Can you work these out from the model? Positions are in its coordinate system, mm. A direction names the side the tool comes from. Give positions to 0.01 mm unless a question says otherwise; leave off trailing zeros. Order: outer loops, then holes, each group sorted by start corner. A loop starts at its lowest first (then second) coordinate and runs counter-clockwise, first axis right, second up.
Item 1: If we mould it in two halves opening along Y, with no side actions, what happens to faces 1 (the flat face through (-47.1, 62, 1)), 2 (the flat face through (39.8, 61.57, 1.48)), 3 (the flat face through (-42, 66.1, 1)), 4 (the flat face through (-71, 3, 1))? For each: +Y half, -Y half, draft (parallel to the pull), parting line (faces both ways), or undercut.
Item 2: I want a section at A-A, the plane x = -69.5. Write out the boundary of the cut face in (y, z), then the cut area to 3 significant figures.
Item 3: Which directions (+Z, -Z, +X, -X, +Y, -Y) give clear straight access to the entire face, cutting with the end or side of a thin tool? Please do faces 5 (the flat face through (-50.2, 61.57, 1.48)), 6 (the flat face through (-56.056, -2.735, 1.479)), 7 (the flat face through (-52.1, 59, 1)).
Item 4: If I drill on line 1 along X through (y, z) = (63, 2.45); line 2 along X through (y, z) = (57.5, 2.75); line 3 along Y through (x, z) = (32, 1), over which ranges is the centre line in solid material (lowest first)?
Item 5: I'm going to push flat-ended pins straight in: pin 1 Ø1.5 at (x, z) = (60, 1) entering from -Y; pin 2 Ø8 at (x, y) = (-14, 10.5) entering from -Z; pin 3 Ø1.5 at (y, z) = (2, 1.5) entering from -X; pin 4 Ø0.9 at (y, z) = (2, 1.5) entering from +X. Where does each tip first touch, or does it pass through?
```python
from build123d import *

# Parameters (mm, degrees)
SKETCH1_W            = 162.421633227
SKETCH1_H            = 57
BOSS_EXTRUDE1_DEPTH  = 3
BOTTOM_HOOKS_DEPTH   = 3
TOP_TABS_DEPTH       = 3
TOP_TAB_RELIEF_REACH = 107.556


with BuildPart() as part:
    # Sketch1 → Boss-Extrude1 (new body)
    with BuildSketch(Plane.XY):
        with Locations((-1.032340883, 31.5)):
            Rectangle(SKETCH1_W, SKETCH1_H)
    extrude(amount=BOSS_EXTRUDE1_DEPTH)

    # Sketch2 → bottom hooks (add)
    with BuildSketch(Plane(origin=(0, 0, 0), x_dir=(-1, 0, 0), z_dir=(0, 0, -1))):
        Polygon((52, 3), (60, 3), (60, -0.2), (63, -0.2), (63, -2.2), (65, -2.2), (65, -5.2), (60, -5.2), (52, -0.2), align=None)
        Polygon((-53, -2.2), (-55, -2.2), (-55, -5.2), (-45, -5.2), (-42, -3.2), (-42, -0.2), (-45, -0.2), (-45, 3), (-53, 3), align=None)
    extrude(amount=-BOTTOM_HOOKS_DEPTH)

    # Sketch3 → top tabs (add)
    with BuildSketch(Plane(origin=(0, 0, 0), x_dir=(-1, 0, 0), z_dir=(0, 0, -1))):
        with BuildLine():
            Line((-39.7, 63.1), (-39.9, 60))
            Line((-39.9, 60), (-39.9, 57.1))
            ThreePointArc((-39.9, 57.1), (-38.9, 56.1), (-37.9, 57.1))
            Line((-37.9, 57.1), (-37.9, 60))
            Line((-37.9, 60), (-35.9, 60))
            Line((-35.9, 60), (-35.9, 53))
            Line((-35.9, 53), (-52.1, 53))
            Line((-52.1, 53), (-52.1, 60))
            Line((-52.1, 60), (-50.1, 60))
            Line((-50.1, 60), (-50.1, 63.1))
            Line((-50.1, 63.1), (-50.6, 63.1))
            Line((-50.6, 63.1), (-50.1, 66.1))
            Line((-50.1, 66.1), (-44.9, 66.1))
            Line((-44.9, 66.1), (-44.9, 57.1))
            ThreePointArc((-44.9, 57.1), (-43.9, 56.1), (-42.9, 57.1))
            Line((-42.9, 57.1), (-42.9, 66.1))
            Line((-42.9, 66.1), (-39.7, 66.1))
            Line((-39.7, 66.1), (-39.2, 63.1))
            Line((-39.2, 63.1), (-39.7, 63.1))
        make_face()
        with BuildLine():
            Line((50.3, 63.1), (50.1, 60))
            Line((50.1, 60), (50.1, 57.1))
            ThreePointArc((50.1, 57.1), (51.1, 56.1), (52.1, 57.1))
            Line((52.1, 57.1), (52.1, 60))
            Line((52.1, 60), (54.1, 60))
            Line((54.1, 60), (54.1, 53))
            Line((54.1, 53), (37.9, 53))
            Line((37.9, 53), (37.9, 60))
            Line((37.9, 60), (39.9, 60))
            Line((39.9, 60), (39.9, 63.1))
            Line((39.9, 63.1), (39.4, 63.1))
            Line((39.4, 63.1), (39.9, 66.1))
            Line((39.9, 66.1), (45.1, 66.1))
            Line((45.1, 66.1), (45.1, 57.1))
            ThreePointArc((45.1, 57.1), (46.1, 56.1), (47.1, 57.1))
            Line((47.1, 57.1), (47.1, 66.1))
            Line((47.1, 66.1), (50.3, 66.1))
            Line((50.3, 66.1), (50.8, 63.1))
            Line((50.8, 63.1), (50.3, 63.1))
        make_face()
    extrude(amount=-TOP_TABS_DEPTH)

    # Sketch4 → top tab relief (cut, up to next)
    with BuildSketch(Plane(origin=(0, 0, 0), x_dir=(-1, 0, 0), z_dir=(0, 0, -1)), mode=Mode.PRIVATE) as top_tab_relief_sk1:
        with BuildLine():
            Line((47.1, 57.1), (47.1, 66.1))
            Line((47.1, 66.1), (45.1, 66.1))
            Line((45.1, 66.1), (45.1, 57.1))
            ThreePointArc((45.1, 57.1), (46.1, 56.1), (47.1, 57.1))
        make_face()
    top_tab_relief_tool1 = extrude(top_tab_relief_sk1.sketch, amount=-TOP_TAB_RELIEF_REACH, mode=Mode.PRIVATE) & part.part
    # Sketch4 → top tab relief (cut, up to next)
    with BuildSketch(Plane(origin=(0, 0, 0), x_dir=(-1, 0, 0), z_dir=(0, 0, -1)), mode=Mode.PRIVATE) as top_tab_relief_sk2:
        with BuildLine():
            Line((50.1, 60), (50.1, 57.1))
            ThreePointArc((50.1, 57.1), (51.1, 56.1), (52.1, 57.1))
            Line((52.1, 57.1), (52.1, 60))
            Line((52.1, 60), (50.1, 60))
        make_face()
    top_tab_relief_tool2 = extrude(top_tab_relief_sk2.sketch, amount=-TOP_TAB_RELIEF_REACH, mode=Mode.PRIVATE) & part.part
    # Sketch4 → top tab relief (cut, up to next)
    with BuildSketch(Plane(origin=(0, 0, 0), x_dir=(-1, 0, 0), z_dir=(0, 0, -1)), mode=Mode.PRIVATE) as top_tab_relief_sk3:
        with BuildLine():
            Line((-44.9, 66.1), (-44.9, 57.1))
            ThreePointArc((-44.9, 57.1), (-43.9, 56.1), (-42.9, 57.1))
            Line((-42.9, 57.1), (-42.9, 66.1))
            Line((-42.9, 66.1), (-44.9, 66.1))
        make_face()
    top_tab_relief_tool3 = extrude(top_tab_relief_sk3.sketch, amount=-TOP_TAB_RELIEF_REACH, mode=Mode.PRIVATE) & part.part
    # Sketch4 → top tab relief (cut, up to next)
    with BuildSketch(Plane(origin=(0, 0, 0), x_dir=(-1, 0, 0), z_dir=(0, 0, -1)), mode=Mode.PRIVATE) as top_tab_relief_sk4:
        with BuildLine():
            Line((-39.9, 60), (-39.9, 57.1))
            ThreePointArc((-39.9, 57.1), (-38.9, 56.1), (-37.9, 57.1))
            Line((-37.9, 57.1), (-37.9, 60))
            Line((-37.9, 60), (-39.9, 60))
        make_face()
    top_tab_relief_tool4 = extrude(top_tab_relief_sk4.sketch, amount=-TOP_TAB_RELIEF_REACH, mode=Mode.PRIVATE) & part.part
    add(top_tab_relief_tool1.solids().sort_by_distance((-46.1, 61.204755, 0))[0], mode=Mode.SUBTRACT)
    add(top_tab_relief_tool2.solids().sort_by_distance((-51.1, 58.150542, 0))[0], mode=Mode.SUBTRACT)
    add(top_tab_relief_tool3.solids().sort_by_distance((43.9, 61.204755, 0))[0], mode=Mode.SUBTRACT)
    add(top_tab_relief_tool4.solids().sort_by_distance((38.9, 58.150542, 0))[0], mode=Mode.SUBTRACT)


solid = part.part
```
Results list:
1. face 1: draft
1. face 2: undercut
1. face 3: +Y half
1. face 4: undercut
2. outline: (3, 0) - (60, 0) - (60, 3) - (3, 3) - close
2. area: 171 mm2
3. face 5: +Z, -Z, -X
3. face 6: +Z, -Z, -Y
3. face 7: +Z, -Z, +Y
4. line 1: x = -50.29 to -47.1, -45.1 to -39.9, 39.71 to 42.9, 44.9 to 50.1
4. line 2: x = -82.24 to -52.1, -50.1 to -47.1, -45.1 to 37.9, 39.9 to 42.9, 44.9 to 80.18
4. line 3: y = 3 to 60
5. pin 1: stops at y = 3
5. pin 2: stops at z = 0
5. pin 3: stops at x = -60
5. pin 4: stops at x = 53
